Source: CAD feature listing. Evaluate the final solid. Frame: model axes, mm. Face numbers are marked on the shaded views. A direction names the side the tool comes from. Coordinates: 2 decimals unless noted, no trailing zeros. Loops run counter-clockwise (first coordinate to the right, second up) from the corner with the lowest first, then second, coordinate; pieces in that order, holes last.
```python
from build123d import *

# Parameters (mm, degrees)
F1_DEPTH = 80
F2_R     = 5
F3_SIZE  = 1


with BuildPart() as f1:
    # F0 (on Front) → F1 (new body)
    with BuildSketch(Plane.XZ):
        Polygon((-1.25, 0), (0, 0), (1.25, 0), (2.5, -13.436909), (8.75, -13.436909), (8.75, -53.436909), (28.75, -53.436909), (28.75, 6.563091), (28.75, 20), (19.475808, 20), (0, 20), (-19.475808, 20), (-28.75, 20), (-28.75, 6.563091), (-28.75, -53.436909), (-8.75, -53.436909), (-8.75, -13.436909), (-2.5, -13.436909), align=None)
    extrude(amount=F1_DEPTH)

    # F2
    f2_edges = [f1.edges().sort_by_distance(p)[0] for p in [
        (28.75, -80, -16.718455),
        (-28.75, -80, -16.718455),
        (28.75, 0, -16.718455),
        (-8.75, -40, -53.436909),
        (8.75, -40, -53.436909),
        (-28.75, 0, -16.718455),
    ]]
    fillet(f2_edges, radius=F2_R)

    # F3
    f3_edges = [f1.edges().sort_by_distance(p)[0] for p in [
        (2.5, -40, -13.436909),
        (-2.5, -40, -13.436909),
    ]]
    chamfer(f3_edges, length=F3_SIZE)


solid = f1.part
```
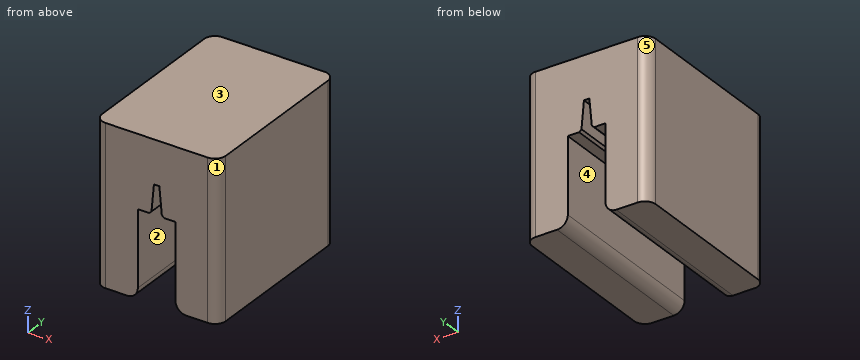
Q1. Section query A-A on z = -22. Return the cut outline in (x, y), then the cut area to 3 significant figures.
Q2. Section query D-D on z = -11. Return the cut outline in (x, y).
Q3. Draft query along X for the marked faces 1, 2 and 3. Return one class per face: released by +X, released by -X, zero draft, split by the parting line, or undercut.
Q4. First-contact query: pin 1 Ø4 at (x, y) = (7.5, -36) entering from -Z; pin 2 Ø1.6 at (x, y) = (-7, -46) entering from -Z. Flat tips, straight axial feed; report the tip coordinate or a pass-through.
Q5. Reachability of the marked faces 4 and 5 from +Z, -Z, +X, -X, +Y, -Y: full face, straight path, thin tool, end or side. Return the list, or none.
Q6. Section query B-B on y = -72. Return the cut outline in (x, z).
Q7. Material intervals for line 1 along X through (y, z) = (-22.5, -39); line 2 along Z through (x, y) = (-8.5, -68.5); line 3 along X through (y, z) = (-74.5, -12), sorted ascending.
Q8. Section query C-C on x = 6. Return the cut outline in (y, z), then the cut area to 3 significant figures.
Resolved:
1. outline: (-28.75, -75) arc R5 ccw to (-23.75, -80) - (-8.75, -80) - (-8.75, 0) - (-23.75, 0) arc R5 ccw to (-28.75, -5) - close; (8.75, -80) - (23.75, -80) arc R5 ccw to (28.75, -75) - (28.75, -5) arc R5 ccw to (23.75, 0) - (8.75, 0) - close
1. area: 3,180 mm2
2. outline: (-28.75, -75) arc R5 ccw to (-23.75, -80) - (-2.27, -80) - (-2.27, 0) - (-23.75, 0) arc R5 ccw to (-28.75, -5) - close; (2.27, -80) - (23.75, -80) arc R5 ccw to (28.75, -75) - (28.75, -5) arc R5 ccw to (23.75, 0) - (2.27, 0) - close
3. face 1: released by +X
3. face 2: undercut
3. face 3: zero draft
4. pin 1: stops at z = -51.07
4. pin 2: stops at z = -13.44
5. face 4: -Z, +Y, -Y
5. face 5: +Z, -Z, -X, +Y
6. outline: (-28.75, -53.44) - (-13.75, -53.44) arc R5 ccw to (-8.75, -48.44) - (-8.75, -13.44) - (-3.5, -13.44) - (-2.41, -12.44) - (-1.25, 0) - (1.25, 0) - (2.41, -12.44) - (3.5, -13.44) - (8.75, -13.44) - (8.75, -48.44) arc R5 ccw to (13.75, -53.44) - (28.75, -53.44) - (28.75, 20) - (-28.75, 20) - close
7. line 1: x = -28.75 to -8.75, 8.75 to 28.75
7. line 2: z = -13.44 to 20
7. line 3: x = -28.75 to -2.37, 2.37 to 28.75
8. outline: (-80, -13.44) - (0, -13.44) - (0, 20) - (-80, 20) - close
8. area: 2,670 mm2
